Here's how the part is built. I have some questions about the finished solid (model axes, mm). A direction names the side the tool comes from. Coordinates: 2 decimals unless noted, no trailing zeros. Write each loop counter-clockwise with the first axis right and the second up, starting at its lowest first coordinate (ties: lowest second). Pieces come first, ordered by that corner, then holes. Notation, with made-up numbers: M 33,73 L 48,73 A24 cw 48,112 Z; hole C 27.5,-9.5 d3. An arc over 180 degrees is marked long. Use a Markdown table: item, result.
```python
from build123d import *

# Parameters (mm, degrees)
F0_W     = 215.9
F0_H     = 279.4
F1_DEPTH = 25.4


with BuildPart() as f1:
    # F0 (on Top) → F1 (new body)
    with BuildSketch(Plane.XY):
        Rectangle(F0_W, F0_H)
        with BuildLine():
            Line((-95.25, -120.65), (-95.25, 120.65))
            ThreePointArc((-95.25, 120.65), (-93.390128, 125.140128), (-88.9, 127))
            Line((-88.9, 127), (-50.670538, 127))
            ThreePointArc((-50.670538, 127), (-47.028327, 125.851615), (-44.703489, 122.821828))
            Line((-44.703489, 122.821828), (0, 0))
            Line((0, 0), (44.703489, 122.821828))
            ThreePointArc((44.703489, 122.821828), (47.028327, 125.851615), (50.670538, 127))
            Line((50.670538, 127), (88.9, 127))
            ThreePointArc((88.9, 127), (93.390128, 125.140128), (95.25, 120.65))
            Line((95.25, 120.65), (95.25, -120.65))
            ThreePointArc((95.25, -120.65), (93.390128, -125.140128), (88.9, -127))
            Line((88.9, -127), (57.15, -127))
            ThreePointArc((57.15, -127), (52.659872, -125.140128), (50.8, -120.65))
            Line((50.8, -120.65), (50.8, 9.608747))
            Line((50.8, 9.608747), (21.034386, -72.171606))
            ThreePointArc((21.034386, -72.171606), (18.709548, -75.201393), (15.067338, -76.349778))
            Line((15.067338, -76.349778), (0, -76.349778))
            Line((0, -76.349778), (-15.067338, -76.349778))
            ThreePointArc((-15.067338, -76.349778), (-18.709548, -75.201393), (-21.034386, -72.171606))
            Line((-21.034386, -72.171606), (-50.8, 9.608747))
            Line((-50.8, 9.608747), (-50.8, -120.65))
            ThreePointArc((-50.8, -120.65), (-52.659872, -125.140128), (-57.15, -127))
            Line((-57.15, -127), (-88.9, -127))
            ThreePointArc((-88.9, -127), (-93.390128, -125.140128), (-95.25, -120.65))
        make_face(mode=Mode.SUBTRACT)
    extrude(amount=F1_DEPTH)


solid = f1.part
```
1. I need wall thicknesses on probe 1 along X at (y, z) = (-114, 3.5); probe 2 along Y at (x, z) = (-76.5, 21.75); probe 3 along X at (y, z) = (70.5, 4.25). Which ranges of each line are inside material? Lowest first, please.
Answers follow:
| item | result |
|---|---|
| probe 1 | x = -107.95 to -95.25, -50.8 to 50.8, 95.25 to 107.95 |
| probe 2 | y = -139.7 to -127, 127 to 139.7 |
| probe 3 | x = -107.95 to -95.25, -25.66 to 25.66, 95.25 to 107.95 |
2. Which directions (+Z, -Z, +X, -X, +Y, -Y) give clear straight access to the entire face, cutting with the end or side of a thin tool? Please do faces 5 (the face through (107.95, -2, 13)), 6 (the face through (18.754, -75.17, 12.522)).
Answers follow:
| item | result |
|---|---|
| face 5 | +Z, -Z, +X, +Y, -Y |
| face 6 | +Z, -Z |
3. Suppose I cut it at A-A on y = -96. Write out the boundary of the cut face in (x, z), and give its area (3 significant figures).
Answers follow:
| item | result |
|---|---|
| outline | M -107.95,0 L -95.25,0 L -95.25,25.4 L -107.95,25.4 Z; M -50.8,0 L 50.8,0 L 50.8,25.4 L -50.8,25.4 Z; M 95.25,0 L 107.95,0 L 107.95,25.4 L 95.25,25.4 Z |
| area | 3,230 mm2 |
4. We'd pull the mould along Y, two halves only. Please class faces 1 (the face through (-2, 139.7, 13)), 2 (the face through (-107.95, -2, 13)), 3 (the face through (52.71, -125.19, 12.52)), 4 (the face through (-52.61, -125.09, 12.52)): +Y half, -Y half, draft (parallel to the pull), parting line (faces both ways), or undercut.
Answers follow:
| item | result |
|---|---|
| face 1 | +Y half |
| face 2 | draft |
| face 3 | undercut |
| face 4 | undercut |
5. Suppose I cut it at D-D on y = -3. Write out the boundary of the cut face in (x, z).
Answers follow:
| item | result |
|---|---|
| outline | M -107.95,0 L -95.25,0 L -95.25,25.4 L -107.95,25.4 Z; M -50.8,0 L -46.21,0 L -46.21,25.4 L -50.8,25.4 Z; M 46.21,0 L 50.8,0 L 50.8,25.4 L 46.21,25.4 Z; M 95.25,0 L 107.95,0 L 107.95,25.4 L 95.25,25.4 Z |
6. Suppose I cut it at C-C on z = 6. Write out the boundary of the cut face in (x, y), and give its area (3 significant figures).
Answers follow:
| item | result |
|---|---|
| outline | M -107.95,-139.7 L 107.95,-139.7 L 107.95,139.7 L -107.95,139.7 Z; hole M -95.25,-120.65 A6.35 ccw -88.9,-127 L -57.15,-127 A6.35 ccw -50.8,-120.65 L -50.8,9.61 L -21.03,-72.17 A6.35 ccw -15.07,-76.35 L 15.07,-76.35 A6.35 ccw 21.03,-72.17 L 50.8,9.61 L 50.8,-120.65 A6.35 ccw 57.15,-127 L 88.9,-127 A6.35 ccw 95.25,-120.65 L 95.25,120.65 A6.35 ccw 88.9,127 L 50.67,127 A6.35 ccw 44.7,122.82 L 0,0 L -44.7,122.82 A6.35 ccw -50.67,127 L -88.9,127 A6.35 ccw -95.25,120.65 Z |
| area | 25,700 mm2 |
7. Suppose I cut it at B-B on x = 73.5. Write out the boundary of the cut face in (y, z), and give its area (3 significant figures).
Answers follow:
| item | result |
|---|---|
| outline | M -139.7,0 L -127,0 L -127,25.4 L -139.7,25.4 Z; M 127,0 L 139.7,0 L 139.7,25.4 L 127,25.4 Z |
| area | 645 mm2 |
